```python
from build123d import *

# Parameters (mm, degrees)
SKETCH1_W           = 74
SKETCH1_H           = 50
BOSS_EXTRUDE1_DEPTH = 30
SKETCH2_R           = 10.5
CUT_EXTRUDE1_DEPTH  = 10
SKETCH3_R           = 6.25
CUT_EXTRUDE2_DEPTH  = 10
SKETCH4_W           = 7
SKETCH4_H           = 20
CUT_EXTRUDE3_DEPTH  = 111
SKETCH5_W           = 7
SKETCH5_H           = 18
SKETCH5_W_2         = 9
CUT_EXTRUDE4_DEPTH  = 111
SKETCH6_R           = 1.65
CUT_EXTRUDE5_DEPTH  = 111
SKETCH7_W           = 74
SKETCH7_H           = 5
BOSS_EXTRUDE2_DEPTH = 45
SKETCH8_W           = 25
SKETCH8_H           = 5
BOSS_EXTRUDE3_DEPTH = 15
SKETCH9_W           = 25
SKETCH9_H           = 5
BOSS_EXTRUDE4_DEPTH = 15
SKETCH10_R          = 6
CUT_EXTRUDE6_DEPTH  = 50
FILLET1_R           = 1


with BuildPart() as part:
    # Sketch1 → Boss-Extrude1 (new body)
    with BuildSketch(Plane.XY):
        with Locations((37, 25)):
            Rectangle(SKETCH1_W, SKETCH1_H)
    extrude(amount=BOSS_EXTRUDE1_DEPTH)

    # Sketch2 → Cut-Extrude1 (cut)
    with BuildSketch(Plane.XZ):
        with Locations((12.74, 15)):
            Circle(SKETCH2_R)
        with Locations((61.26167258, 15)):
            Circle(SKETCH2_R)
    extrude(amount=-CUT_EXTRUDE1_DEPTH, mode=Mode.SUBTRACT)

    # Sketch3 → Cut-Extrude2 (cut)
    with BuildSketch(Plane.XZ.offset(-10)):
        with Locations((12.74, 15)):
            Circle(SKETCH3_R)
        with Locations((61.26167258, 15)):
            Circle(SKETCH3_R)
    extrude(amount=-CUT_EXTRUDE2_DEPTH, mode=Mode.SUBTRACT)

    # Sketch4 → Cut-Extrude3 (cut)
    with BuildSketch(Plane.ZY):
        with Locations((15.5, 40)):
            Rectangle(SKETCH4_W, SKETCH4_H)
    extrude(amount=-CUT_EXTRUDE3_DEPTH, mode=Mode.SUBTRACT)

    # Sketch5 → Cut-Extrude4 (cut)
    with BuildSketch(Plane(origin=(74, 0, 0), x_dir=(0, 0, -1), z_dir=(1, 0, 0))):
        with Locations((-26.5, 41)):
            Rectangle(SKETCH5_W, SKETCH5_H)
        with Locations((-4.5, 41)):
            Rectangle(SKETCH5_W_2, SKETCH5_H)
    extrude(amount=-CUT_EXTRUDE4_DEPTH, mode=Mode.SUBTRACT)

    # Sketch6 → Cut-Extrude5 (cut)
    with BuildSketch(Plane(origin=(0, 0, 9), x_dir=(-1, 0, 0), z_dir=(0, 0, -1))):
        with Locations((-62, 38.308927031)):
            Circle(SKETCH6_R)
        with Locations((-12, 38.308927031)):
            Circle(SKETCH6_R)
    extrude(amount=-CUT_EXTRUDE5_DEPTH, mode=Mode.SUBTRACT)

    # Sketch7 → Boss-Extrude2 (add)
    with BuildSketch(Plane(origin=(0, 0, 0), x_dir=(-1, 0, 0), z_dir=(0, 0, -1))):
        with Locations((-37, 11.5)):
            Rectangle(SKETCH7_W, SKETCH7_H)
    extrude(amount=BOSS_EXTRUDE2_DEPTH)

    # Sketch8 → Boss-Extrude3 (add)
    with BuildSketch(Plane(origin=(74, 0, 0), x_dir=(0, 0, -1), z_dir=(1, 0, 0))):
        with Locations((32.5, 11.5)):
            Rectangle(SKETCH8_W, SKETCH8_H)
    extrude(amount=BOSS_EXTRUDE3_DEPTH)

    # Sketch9 → Boss-Extrude4 (add)
    with BuildSketch(Plane.ZY):
        with Locations((-32.5, 11.5)):
            Rectangle(SKETCH9_W, SKETCH9_H)
    extrude(amount=BOSS_EXTRUDE4_DEPTH)

    # Sketch10 → Cut-Extrude6 (cut)
    with BuildSketch(Plane.XZ):
        with Locations((-2.254021422, -31.146852886)):
            Circle(SKETCH10_R)
        with Locations((76.255693998, -31.146852886)):
            Circle(SKETCH10_R)
    extrude(amount=-CUT_EXTRUDE6_DEPTH, mode=Mode.SUBTRACT)

    # Fillet1
    fillet1_edges = [part.edges().sort_by_distance(p)[0] for p in [
        (74, 11.5, -20),
        (89, 11.5, -45),
        (89, 11.5, -20),
        (0, 11.5, -20),
        (-15, 11.5, -45),
        (-15, 11.5, -20),
    ]]
    fillet(fillet1_edges, radius=FILLET1_R)


solid = part.part
```
Source: CAD feature listing. Evaluate the final solid. Frame: model axes, mm. A direction names the side the tool comes from. Give positions to 0.01 mm unless a question says otherwise; leave off trailing zeros. Loops run counter-clockwise (first coordinate to the right, second up) from the corner with the lowest first, then second, coordinate; pieces in that order, holes last. Notation, with made-up numbers: (-29, -1) -> (11, -1) arc R18 ccw to (11, 15) -> close; hole circle Ø2 at (8, 33.5). An arc over 180 degrees is marked (long way). Put each result on its own line as item: value. Start each with the question number.
1) Material intervals for probe 1 along Y at (x, z) = (62, 10); probe 2 along Z at (x, y) = (30, 30.5); probe 3 along Z at (x, y) = (12.74, 5), sorted ascending.
2) Cut plane D-D (x = 33). Return loops of the section in (y, z).
3) Cut plane B-B (z = 15). Return loops of the section in (x, y).
4) Reachability of faces 1 (the face through (38, 9, -23)), 2 (the face through (36, 16, 30)), 3 (the face through (0, 19, 16)), 4 (the face through (61, 20, 15)) from +Z, -Z, +X, -X, +Y, -Y: full face, straight path, thin tool, end or side. Return the list, or none.
5) Cut plane C-C (x = 12). State how many separate pieces and enclosed holes the cut face has, then the cut area to 3 significant figures.
6) Draft query along X for faces 5 (the face through (38, 32, 27)), 6 (the face through (-15, 12, -33)), 7 (the face through (8.13, 14.93, 19.22)). Return one class per face: released by +X, released by -X, zero draft, split by the parting line, or undercut.
7) Contact query for flat-ended pins moving along their axis: P1, Ø6, axis at x = 61.5, z = 13.5, coming from the -Y side; P2, Ø22.5, axis at x = 59.5, z = -23.5, coming from the +Y side; P3, Ø2.5, axis at x = 34.5, z = 2.5, coming from the +Y side. Output: stop coordinate, or through.
8) Cut plane A-A (x = 81). Return loops of the section in (y, z).
Results are:
1. probe 1: y = 20 to 36.66, 39.96 to 50
1. probe 2: z = 0 to 12, 19 to 30
1. probe 3: z = 0 to 4.5, 25.5 to 30
2. outline: (0, 0) -> (9, 0) -> (9, -45) -> (14, -45) -> (14, 0) -> (32, 0) -> (32, 9) -> (50, 9) -> (50, 12) -> (30, 12) -> (30, 19) -> (50, 19) -> (50, 23) -> (32, 23) -> (32, 30) -> (0, 30) -> close
3. outline: (0, 0) -> (2.24, 0) -> (2.24, 10) -> (6.49, 10) -> (6.49, 20) -> (18.99, 20) -> (18.99, 10) -> (23.24, 10) -> (23.24, 0) -> (50.76, 0) -> (50.76, 10) -> (55.01, 10) -> (55.01, 20) -> (67.51, 20) -> (67.51, 10) -> (71.76, 10) -> (71.76, 0) -> (74, 0) -> (74, 30) -> (0, 30) -> close
4. face 1: -Z, +X, -X, -Y
4. face 2: +Z, +X, -X, +Y, -Y
4. face 3: +Z, -X, +Y, -Y
4. face 4: -Y
5. separate pieces: 3
5. enclosed holes: 0
5. area: 940 mm2
6. face 5: zero draft
6. face 6: released by -X
6. face 7: undercut
7. P1: stops at y = 20
7. P2: stops at y = 14
7. P3: stops at y = 32
8. outline: (9, -45) -> (14, -45) -> (14, -34.82) -> (9, -34.82) -> close; (9, -27.47) -> (14, -27.47) -> (14, -20) -> (9, -20) -> close
